Geometry check sheet. Reference: the model listing, model coordinates, mm. A direction names the side the tool comes from. Give positions to 0.01 mm unless a question says otherwise; leave off trailing zeros. Loops run counter-clockwise (first coordinate to the right, second up) from the corner with the lowest first, then second, coordinate; pieces in that order, holes last. Notation, with made-up numbers: (-20, -12) -> (19, -12) arc R21 cw to (19, 24) -> close; hole circle Ø1 at (35, 21.25). An arc over 180 degrees is marked (long way). Write item = value, one per line.
```python
from build123d import *

# Parameters (mm, degrees)
F0_R     = 30
F0_R_2   = 15
F1_DEPTH = 5
F2_DEPTH = 25


with BuildPart() as f1:
    # F0 (on Front) → F1 (new body)
    with BuildSketch(Plane.XZ):
        Circle(F0_R)
        Circle(F0_R_2, mode=Mode.SUBTRACT)
    extrude(amount=F1_DEPTH)

    # F3 (on face) → F2 (cut)
    with BuildSketch(Plane.XZ.offset(5)):
        with BuildLine():
            ThreePointArc((7.5, 29.0473750966), (3.7801287745, 29.760890888), (0, 30))
            Line((0, 30), (0, 27))
            Line((0, 27), (7.5, 27))
            Line((7.5, 27), (7.5, 29.0473750966))
        make_face()
        with BuildLine():
            Line((0, 27), (0, 30))
            ThreePointArc((0, 30), (-3.7801287745, 29.760890888), (-7.5, 29.0473750966))
            Line((-7.5, 29.0473750966), (-7.5, 27))
            Line((-7.5, 27), (0, 27))
        make_face()
        with BuildLine():
            Line((-17.6335575688, 24.2705098312), (-15.8702018119, 21.8434588481))
            Line((-15.8702018119, 21.8434588481), (-9.8025743541, 26.2518482403))
            Line((-9.8025743541, 26.2518482403), (-11.0059912418, 27.9082094873))
            ThreePointArc((-11.0059912418, 27.9082094873), (-14.4348243396, 26.2989704415), (-17.6335575688, 24.2705098312))
        make_face()
        with BuildLine():
            Line((-21.9378292697, 17.4350694559), (-15.8702018119, 21.8434588481))
            Line((-15.8702018119, 21.8434588481), (-17.6335575688, 24.2705098312))
            ThreePointArc((-17.6335575688, 24.2705098312), (-20.5512011785, 21.8551625507), (-23.1412461574, 19.0914307029))
            Line((-23.1412461574, 19.0914307029), (-21.9378292697, 17.4350694559))
        make_face()
        with BuildLine():
            Line((-28.5316954889, 9.2705098312), (-25.67852594, 8.3434588481))
            Line((-25.67852594, 8.3434588481), (-23.3608984822, 15.4763827203))
            Line((-23.3608984822, 15.4763827203), (-25.308067909, 16.109056419))
            ThreePointArc((-25.308067909, 16.109056419), (-27.1361651776, 12.7917371555), (-28.5316954889, 9.2705098312))
        make_face()
        with BuildLine():
            Line((-27.9961533978, 1.2105349759), (-25.67852594, 8.3434588481))
            Line((-25.67852594, 8.3434588481), (-28.5316954889, 9.2705098312))
            ThreePointArc((-28.5316954889, 9.2705098312), (-29.472413242, 5.6015049487), (-29.9433228247, 1.8432086746))
            Line((-29.9433228247, 1.8432086746), (-27.9961533978, 1.2105349759))
        make_face()
        with BuildLine():
            Line((-28.5316954889, -9.2705098312), (-25.67852594, -8.3434588481))
            Line((-25.67852594, -8.3434588481), (-27.9961533978, -1.2105349759))
            Line((-27.9961533978, -1.2105349759), (-29.9433228247, -1.8432086746))
            ThreePointArc((-29.9433228247, -1.8432086746), (-29.472413242, -5.6015049487), (-28.5316954889, -9.2705098312))
        make_face()
        with BuildLine():
            Line((-23.3608984822, -15.4763827203), (-25.67852594, -8.3434588481))
            Line((-25.67852594, -8.3434588481), (-28.5316954889, -9.2705098312))
            ThreePointArc((-28.5316954889, -9.2705098312), (-27.1361651776, -12.7917371555), (-25.308067909, -16.109056419))
            Line((-25.308067909, -16.109056419), (-23.3608984822, -15.4763827203))
        make_face()
        with BuildLine():
            Line((-17.6335575688, -24.2705098312), (-15.8702018119, -21.8434588481))
            Line((-15.8702018119, -21.8434588481), (-21.9378292697, -17.4350694559))
            Line((-21.9378292697, -17.4350694559), (-23.1412461574, -19.0914307029))
            ThreePointArc((-23.1412461574, -19.0914307029), (-20.5512011785, -21.8551625507), (-17.6335575688, -24.2705098312))
        make_face()
        with BuildLine():
            Line((-9.8025743541, -26.2518482403), (-15.8702018119, -21.8434588481))
            Line((-15.8702018119, -21.8434588481), (-17.6335575688, -24.2705098312))
            ThreePointArc((-17.6335575688, -24.2705098312), (-14.4348243396, -26.2989704415), (-11.0059912418, -27.9082094873))
            Line((-11.0059912418, -27.9082094873), (-9.8025743541, -26.2518482403))
        make_face()
        with BuildLine():
            Line((0, -30), (0, -27))
            Line((0, -27), (-7.5, -27))
            Line((-7.5, -27), (-7.5, -29.0473750966))
            ThreePointArc((-7.5, -29.0473750966), (-3.7801287745, -29.760890888), (0, -30))
        make_face()
        with BuildLine():
            Line((7.5, -27), (0, -27))
            Line((0, -27), (0, -30))
            ThreePointArc((0, -30), (3.7801287745, -29.760890888), (7.5, -29.0473750966))
            Line((7.5, -29.0473750966), (7.5, -27))
        make_face()
        with BuildLine():
            Line((17.6335575688, -24.2705098312), (15.8702018119, -21.8434588481))
            Line((15.8702018119, -21.8434588481), (9.8025743541, -26.2518482403))
            Line((9.8025743541, -26.2518482403), (11.0059912418, -27.9082094873))
            ThreePointArc((11.0059912418, -27.9082094873), (14.4348243396, -26.2989704415), (17.6335575688, -24.2705098312))
        make_face()
        with BuildLine():
            Line((21.9378292697, -17.4350694559), (15.8702018119, -21.8434588481))
            Line((15.8702018119, -21.8434588481), (17.6335575688, -24.2705098312))
            ThreePointArc((17.6335575688, -24.2705098312), (20.5512011785, -21.8551625507), (23.1412461574, -19.0914307029))
            Line((23.1412461574, -19.0914307029), (21.9378292697, -17.4350694559))
        make_face()
        with BuildLine():
            Line((28.5316954889, -9.2705098312), (25.67852594, -8.3434588481))
            Line((25.67852594, -8.3434588481), (23.3608984822, -15.4763827203))
            Line((23.3608984822, -15.4763827203), (25.308067909, -16.109056419))
            ThreePointArc((25.308067909, -16.109056419), (27.1361651776, -12.7917371555), (28.5316954889, -9.2705098312))
        make_face()
        with BuildLine():
            Line((27.9961533978, -1.2105349759), (25.67852594, -8.3434588481))
            Line((25.67852594, -8.3434588481), (28.5316954889, -9.2705098312))
            ThreePointArc((28.5316954889, -9.2705098312), (29.472413242, -5.6015049487), (29.9433228247, -1.8432086746))
            Line((29.9433228247, -1.8432086746), (27.9961533978, -1.2105349759))
        make_face()
        with BuildLine():
            Line((28.5316954889, 9.2705098312), (25.67852594, 8.3434588481))
            Line((25.67852594, 8.3434588481), (27.9961533978, 1.2105349759))
            Line((27.9961533978, 1.2105349759), (29.9433228247, 1.8432086746))
            ThreePointArc((29.9433228247, 1.8432086746), (29.472413242, 5.6015049487), (28.5316954889, 9.2705098312))
        make_face()
        with BuildLine():
            Line((23.3608984822, 15.4763827203), (25.67852594, 8.3434588481))
            Line((25.67852594, 8.3434588481), (28.5316954889, 9.2705098312))
            ThreePointArc((28.5316954889, 9.2705098312), (27.1361651776, 12.7917371555), (25.308067909, 16.109056419))
            Line((25.308067909, 16.109056419), (23.3608984822, 15.4763827203))
        make_face()
        with BuildLine():
            Line((17.6335575688, 24.2705098312), (15.8702018119, 21.8434588481))
            Line((15.8702018119, 21.8434588481), (21.9378292697, 17.4350694559))
            Line((21.9378292697, 17.4350694559), (23.1412461574, 19.0914307029))
            ThreePointArc((23.1412461574, 19.0914307029), (20.5512011785, 21.8551625507), (17.6335575688, 24.2705098312))
        make_face()
        with BuildLine():
            Line((9.8025743541, 26.2518482403), (15.8702018119, 21.8434588481))
            Line((15.8702018119, 21.8434588481), (17.6335575688, 24.2705098312))
            ThreePointArc((17.6335575688, 24.2705098312), (14.4348243396, 26.2989704415), (11.0059912418, 27.9082094873))
            Line((11.0059912418, 27.9082094873), (9.8025743541, 26.2518482403))
        make_face()
    extrude(amount=-F2_DEPTH, mode=Mode.SUBTRACT)


solid = f1.part
```
Item 1: Draft check along Z on faces 6 (the flat face through (25.646, -2.535, 8.443)), 7 (the flat face through (10.396, -2.535, -27.068)), 8 (the cylindrical face through (-9.3, -2.46, -28.52)), 9 (the flat face through (-7.5, -3, -28)). Enter one of: +Z half, -Z half, draft (parallel to the pull), parting line (faces both ways), or undercut.
Answer:
face_6 = undercut
face_7 = undercut
face_8 = -Z half
face_9 = draft
Item 2: Thickness scan on L1, parallel to Z at x = 0, y = -2.35; L2, parallel to X at y = -0.5, z = -5; L3, parallel to X at y = -1.75, z = -12. Record the ranges inside material, lowest first. Write a range as [from, to].
Answer:
L1 = [-27, -15], [15, 27]
L2 = [-26.76, -14.14], [14.14, 26.76]
L3 = [-24.49, -9], [9, 24.49]
Item 3: Section check B-B, the plane x = 0. Record the cut outline in (y, z), plus the area to 3 significant figures.
Answer:
outline = (-5, -27) -> (0, -27) -> (0, -15) -> (-5, -15) -> close; (-5, 15) -> (0, 15) -> (0, 27) -> (-5, 27) -> close
area = 120 mm^2
Item 4: Section check D-D, the plane z = -23. Record the cut outline in (x, y), plus the area to 3 significant figures.
Answer:
outline = (-14.28, -5) -> (14.28, -5) -> (14.28, 0) -> (-14.28, 0) -> close
area = 143 mm^2
Item 5: Tool access check on faces 1 (the cylindrical face through (30, -2, 0)), 2 (the flat face through (-10.396, -2.535, 27.068)), 3 (the cylindrical face through (9.25, -2.46, -28.54)), 4 (the flat face through (0, -3, 27)), 5 (the flat face through (-28.956, -2.535, -1.522)). Record the directions out of +Z, -Z, +X, -X, +Y, -Y that give a thin tool (end or side, any length) a straight path to the whole face; none if there is none.
Answer:
face_1 = +X, +Y, -Y
face_2 = -X, +Y, -Y
face_3 = -Z, +X, +Y, -Y
face_4 = +Z, +Y, -Y
face_5 = -Z, +Y, -Y
Item 6: Section check C-C, the plane x = 18. Record the cut outline in (y, z).
Answer:
outline = (-5, -20.3) -> (0, -20.3) -> (0, 20.3) -> (-5, 20.3) -> close
Item 7: Gauge pin test, flat ends, axial feed: pin 1 (1.5 mm diameter, centred on x = 22.5, y = -3.5, fed in from +Z); pin 2 (1.6 mm diameter, centred on y = -2, z = 27.5, fed in from -X); pin 3 (2.5 mm diameter, centred on x = 2, y = -3, fed in from -Z). Record the tip position at first contact, or that the pin passes through.
Answer:
pin_1 = 19.09
pin_2 = -11.01
pin_3 = -27
Item 8: Section check A-A, the plane z = 0. Record the cut outline in (x, y).
Answer:
outline = (-30, -5) -> (-15, -5) -> (-15, 0) -> (-30, 0) -> close; (15, -5) -> (30, -5) -> (30, 0) -> (15, 0) -> close
